The model under review builds one solid part; all positions refer to its coordinate system, in mm. Round coordinates to 2 decimals unless told otherwise and drop trailing zeros. Order: outer loops, then holes, each group sorted by start corner. A loop starts at its lowest first (then second) coordinate and runs counter-clockwise, first axis right, second up.
```python
from build123d import *

# Parameters (mm, degrees)
EXTRUDE_1_DEPTH   = 2
HOLE_WIZARD_M61_D = 6.5


with BuildPart() as part:
    # Эскиз1 → Вытянуть1 (new body)
    with BuildSketch(Plane.XY):
        Polygon((-70, 48.5), (-70, 57), (70, 57), (70, 48.5), (82, 48.5), (82, -39.5), (70, -39.5), (70, -57), (-70, -57), (-70, -39.5), (-82, -39.5), (-82, 48.5), align=None)
    extrude(amount=EXTRUDE_1_DEPTH)

    # Отверстие с зазором M61 (through all)
    with Locations(Plane(origin=(-76, 27.5, 2), x_dir=(1, 0, 0), z_dir=(0, 0, 1))):
        with Locations((0, 0), (0, -45), (26, -72.5), (76, -72.5), (126, -72.5), (126, 17.5), (76, 17.5), (26, 17.5), (152, 0), (152, -45)):
            Hole(HOLE_WIZARD_M61_D / 2)


solid = part.part
```
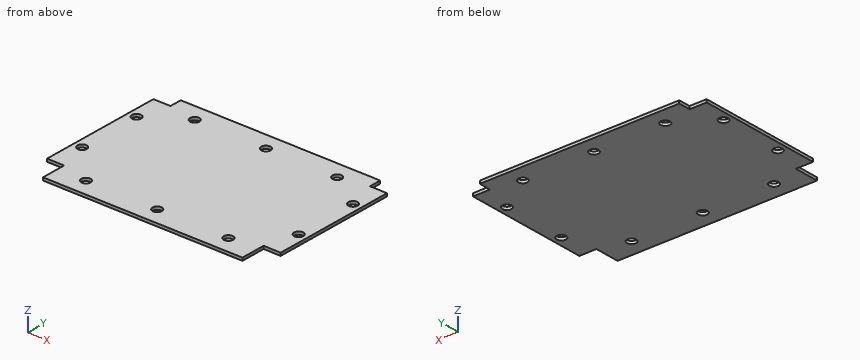
(1) Consider section A-A (y = -45). Write out the cut boundary in (x, z).
Data:
outline: (-70, 0) - (-53.25, 0) - (-53.25, 2) - (-70, 2) - close; (-46.75, 0) - (-3.25, 0) - (-3.25, 2) - (-46.75, 2) - close; (3.25, 0) - (46.75, 0) - (46.75, 2) - (3.25, 2) - close; (53.25, 0) - (70, 0) - (70, 2) - (53.25, 2) - close
(2) Consider section D-D (y = -17.5). Write out the cut boundary in (x, z), and give its area (3 significant figures).
Data:
outline: (-82, 0) - (-79.25, 0) - (-79.25, 2) - (-82, 2) - close; (-72.75, 0) - (72.75, 0) - (72.75, 2) - (-72.75, 2) - close; (79.25, 0) - (82, 0) - (82, 2) - (79.25, 2) - close
area: 302 mm2
(3) To check wall thickness, follow probe 1 along Y at (x, z) = (-76, 1.4); probe 2 along X at (y, z) = (25, 1.5); probe 3 along X at (y, z) = (-16.5, 0.4). State the ranges of each line that lie inside material, in increasing order.
Data:
probe 1: y = -39.5 to -20.75, -14.25 to 24.25, 30.75 to 48.5
probe 2: x = -82 to -78.08, -73.92 to 73.92, 78.08 to 82
probe 3: x = -82 to -79.09, -72.91 to 72.91, 79.09 to 82
(4) Insertion check: pin 1 (1 mm diameter, centred on x = 74.5, z = 0.5, fed in from +Y); pin 2 (0.6 mm diameter, centred on y = 53.5, z = 1, fed in from -X); pin 3 (1 mm diameter, centred on x = -77, z = 1, fed in from -Y). Each pin has a flat end and moves straight along its axis. Give the tip position at first contact, or say it passes through.
Data:
pin 1: stops at y = 48.5
pin 2: stops at x = -70
pin 3: stops at y = -39.5
(5) Consider section C-C (z = 0.5). State how many separate pieces and enclosed holes the cut face has, and give its area (3 significant figures).
Data:
separate pieces: 1
enclosed holes: 10
area: 17,700 mm2
(6) Consider section B-B (x = 76). Write out the cut boundary in (y, z).
Data:
outline: (-39.5, 0) - (-20.75, 0) - (-20.75, 2) - (-39.5, 2) - close; (-14.25, 0) - (24.25, 0) - (24.25, 2) - (-14.25, 2) - close; (30.75, 0) - (48.5, 0) - (48.5, 2) - (30.75, 2) - close
